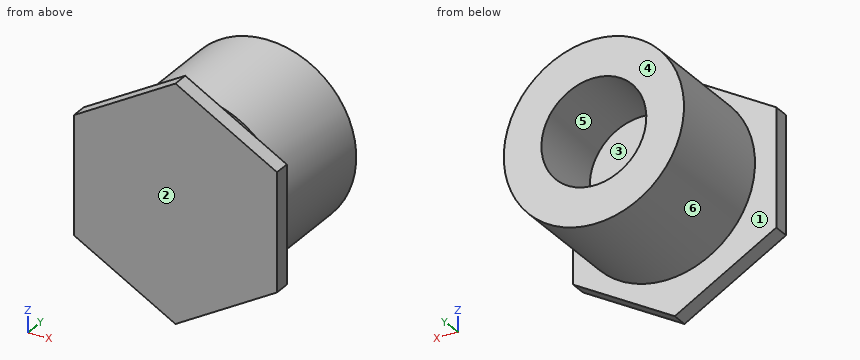
```python
from build123d import *

# Parameters (mm, degrees)
EXTRUDE_1_DEPTH = 0.65


with BuildPart() as part:
    # Эскиз1 → Бобышка-Вытянуть1 (new body)
    with BuildSketch(Plane(origin=(0, 0, 0), x_dir=(1, 0, 0), z_dir=(0, 1, 0))):
        Polygon((0, -4.618802154), (4, -2.309401077), (4, 2.309401077), (0, 4.618802154), (-4, 2.309401077), (-4, -2.309401077), align=None)
    extrude(amount=EXTRUDE_1_DEPTH)

    # Эскиз6 → Повернуть1 (revolve)
    with BuildSketch(Plane.XY, mode=Mode.PRIVATE) as revolve_1_sk:
        Polygon((3.55, 6), (3.55, 1.3), (2.84, 1.3), (2.84, 0.65), (0, 0.65), (0, 2.8), (2.067, 2.8), (2.067, 6), align=None)
    revolve(revolve_1_sk.sketch.rotate(Axis((0, 2.8, 0), (0, -1, 0)), 90), axis=Axis((0, 2.8, 0), (0, -1, 0)))


solid = part.part
```
For this review, take the finished solid that the model builds, in its own axes (mm). Face numbers are marked on the shaded views. A direction names the side the tool comes from. Coordinates: 2 decimals unless noted, no trailing zeros. Order: outer loops, then holes, each group sorted by start corner. A loop starts at its lowest first (then second) coordinate and runs counter-clockwise, first axis right, second up. Notation, with made-up numbers: (30.5, -24.75) - (78.5, -24.75) arc R9 cw to (78.5, -8.75) - close; hole circle Ø11 at (-20, 12.5). An arc over 180 degrees is marked (long way). Answer as a JSON object with one key per item and string values. Group by question number.
1. We need section B-B on x = -3. State the section outline as (y, z) points, then the cut area to 3 significant figures.
2. We need section A-A on z = 0. State the section outline as (x, y) points.
3. We need section C-C on y = 2.45. State the section outline as (x, z) points.
4. We need section D-D on z = 3.25. State the section outline as (x, y) points.
5. For the marked faces 1, 2 and 3, list the 3-axis set-ups (+Z, -Z, +X, -X, +Y, -Y) from which the entire face can be reached by the end or side of a thin tool; tool diameter is ignored.
6. Clearance check with flat-ended pins moving along their axes: P1, Ø1, axis at y = 1, z = -3.5, coming from the -X side; P2, Ø1.2, axis at x = 1, z = 0, coming from the +Y side. State where each tip first meets the part, or that it passes through.
7. The part is to be moulded in two halves that separate along X. For the marked faces 4, 5 and 6, say which applies: pulls with the +X half, pulls with the -X half, needs draft (parallel to the pull), parting line crosses it, or undercut.
8. For probe 1 along X at (y, z) = (4.2, 0); probe 2 along Y at (x, z) = (2.75, 1.25); probe 3 along Y at (x, z) = (-3.5, -0.75), list the stretches that pass through material, from the lowest coordinate up.
Final values:
{
 "1": {"outline": "(0, -2.89) - (0.65, -2.89) - (0.65, 2.89) - (0, 2.89) - close; (1.3, -1.9) - (6, -1.9) - (6, 1.9) - (1.3, 1.9) - close", "area": "21.6 mm²"},
 "2": {"outline": "(-4, 0) - (4, 0) - (4, 0.65) - (2.84, 0.65) - (2.84, 1.3) - (3.55, 1.3) - (3.55, 6) - (2.07, 6) - (2.07, 2.8) - (-2.07, 2.8) - (-2.07, 6) - (-3.55, 6) - (-3.55, 1.3) - (-2.84, 1.3) - (-2.84, 0.65) - (-4, 0.65) - close"},
 "3": {"outline": "circle Ø7.1 at (0, 0)"},
 "4": {"outline": "(-2.37, 0) - (2.37, 0) - (2.37, 0.65) - (-2.37, 0.65) - close; (-1.43, 1.3) - (1.43, 1.3) - (1.43, 6) - (-1.43, 6) - close"},
 "5": {"face 1": "none", "face 2": "+Z, -Z, +X, -X, -Y", "face 3": "+Y"},
 "6": {"P1": "x = -2.56", "P2": "y = 2.8"},
 "7": {"face 4": "needs draft", "face 5": "undercut", "face 6": "parting line crosses it"},
 "8": {"probe 1": "-3.55 to -2.07, 2.07 to 3.55", "probe 2": "0 to 0.65, 1.3 to 6", "probe 3": "0 to 0.65"}
}
